Could you check a few things on this model? Use its own coordinates, in mm. A direction names the side the tool comes from. Round coordinates to 2 decimals unless told otherwise and drop trailing zeros. Order: outer loops, then holes, each group sorted by start corner. A loop starts at its lowest first (then second) coordinate and runs counter-clockwise, first axis right, second up. Notation, with made-up numbers: (78.25, 28.25) - (115.25, 28.25) arc R24 cw to (115.25, 39.25) - close; hole circle Ø1 at (52, -20). An arc over 180 degrees is marked (long way). Use one line per item in the form item = value.
from build123d import *

# Parameters (mm, degrees)
CUT_EXTRUDE1_DEPTH      = 269.763771223
CUT_EXTRUDE1_DEPTH_BACK = 269.763771223
CUT_EXTRUDE4_DEPTH      = 13.97
CUT_EXTRUDE5_DEPTH      = 13.97
CIRPATTERN1_COUNT       = 2
CUT_EXTRUDE6_DEPTH      = 269.763771223
CUT_EXTRUDE6_DEPTH_BACK = 269.763771223
FILLET1_R               = 0.254


with BuildPart() as part:
    # Sketch1 → Revolve1 (revolve)
    with BuildSketch(Plane.XY, mode=Mode.PRIVATE) as revolve1_sk:
        with BuildLine():
            Line((-38.8239, 261.4935178), (-43.9039, 261.4935178))
            Line((-43.9039, 261.4935178), (-43.9039, -38.2264822))
            Line((-43.9039, -38.2264822), (-41.2369, -38.2264822))
            Line((-41.2369, -38.2264822), (-41.2369, -52.1964822))
            Line((-41.2369, -52.1964822), (-36.1569, -52.1964822))
            Line((-36.1569, -52.1964822), (-36.1569, -38.2264822))
            ThreePointArc((-36.1569, -38.2264822), (-36.832638636, -32.406611067), (-38.8239, -26.89640228))
            Line((-38.8239, -26.89640228), (-38.8239, 261.4935178))
        make_face()
    revolve(revolve1_sk.sketch.rotate(Axis((0, 16.071963393, 0), (0, -1, 0)), 270), axis=Axis((0, 16.071963393, 0), (0, -1, 0)))

    # Sketch2 → Cut-Extrude1 (cut, two sides: drawn at the far end of the back side and taken through both)
    with BuildSketch(Plane.XY.offset(-CUT_EXTRUDE1_DEPTH_BACK)):
        with BuildLine():
            Line((-0.771031735, -45.62095313), (0, -45.150169247))
            Line((0, -45.150169247), (0.771031735, -45.62095313))
            ThreePointArc((0.771031735, -45.62095313), (0, -48.363269247), (-0.771031735, -45.62095313))
        make_face()
    extrude(amount=CUT_EXTRUDE1_DEPTH + CUT_EXTRUDE1_DEPTH_BACK, mode=Mode.SUBTRACT)

    # Sketch3 → Cut-Extrude4 (cut)
    with BuildSketch(Plane.XZ.offset(52.1964822)):
        with BuildLine():
            Line((-17.427466998, -37.373323583), (0, 0))
            Line((0, 0), (-17.427466998, 37.373323583))
            ThreePointArc((-17.427466998, 37.373323583), (-41.2369, 0), (-17.427466998, -37.373323583))
        make_face()
        with BuildLine():
            Line((17.427466998, 37.373323583), (0, 0))
            Line((0, 0), (17.427466998, -37.373323583))
            ThreePointArc((17.427466998, -37.373323583), (34.778848712, -22.156570219), (41.2369, 0))
            ThreePointArc((41.2369, 0), (34.778848712, 22.156570219), (17.427466998, 37.373323583))
        make_face()
    extrude(amount=-CUT_EXTRUDE4_DEPTH, mode=Mode.SUBTRACT)

    # Sketch4 → Cut-Extrude5 (cut)
    with BuildSketch(Plane.XZ.offset(52.1964822)):
        with BuildLine():
            ThreePointArc((-3.2004, -41.112520738), (-1.601408002, -41.205793452), (0, -41.2369))
            ThreePointArc((0, -41.2369), (1.601408002, -41.205793452), (3.2004, -41.112520738))
            Line((3.2004, -41.112520738), (-3.2004, -41.112520738))
        make_face()
    cut_extrude5 = extrude(amount=-CUT_EXTRUDE5_DEPTH, mode=Mode.SUBTRACT)

    # CirPattern1: Cut-Extrude5 ×2 about axis
    cirpattern1_axis = Axis((0, 0, 0), (0, 1, 0))
    for i in range(1, CIRPATTERN1_COUNT):
        add(cut_extrude5.rotate(cirpattern1_axis, i * 360 / CIRPATTERN1_COUNT), mode=Mode.SUBTRACT)

    # Sketch5 → Cut-Extrude6 (cut, two sides: drawn at the far end of the back side and taken through both)
    with BuildSketch(Plane.XY.offset(-CUT_EXTRUDE6_DEPTH_BACK)):
        with BuildLine():
            Line((-0.771031735, 258.692283917), (0, 259.1630678))
            Line((0, 259.1630678), (0.771031735, 258.692283917))
            ThreePointArc((0.771031735, 258.692283917), (0, 255.9499678), (-0.771031735, 258.692283917))
        make_face()
    extrude(amount=CUT_EXTRUDE6_DEPTH + CUT_EXTRUDE6_DEPTH_BACK, mode=Mode.SUBTRACT)

    # Fillet1
    fillet1_edges = [part.edges().sort_by_distance(p)[0] for p in [
        (-0.385515867, -45.385561188, 41.112520738),
        (0.385515867, -45.385561188, 41.112520738),
        (0, -48.363269247, 41.112520738),
        (0, -48.363269247, -41.112520738),
        (-0.385515867, -45.385561188, -41.112520738),
        (0.385515867, -45.385561188, -41.112520738),
    ]]
    fillet(fillet1_edges, radius=FILLET1_R)


solid = part.part
Item 1: For faces 1 (the face through (-10.38, -45.31, 39.91)), 2 (the face through (10.38, -45.31, -39.91)), 3 (the face through (-11.66, 119.32, 37.03)), 4 (the face through (-0.221, -43.561, -36.156)), 5 (the face through (-10.582, -45.309, -39.856)), which set-ups out of +Z, -Z, +X, -X, +Y, -Y let a thin tool reach every point of the face, with its end or its side?
Found:
face_1 = +Z, -X, -Y
face_2 = -Z, +X, -Y
face_3 = +Y
face_4 = +Y, -Y
face_5 = -Z, -X, -Y
Item 2: Imagine slicing it at B-B on y = 68. Please give me the cut outline in (x, z).
Found:
outline = circle Ø87.81 at (0, 0); hole circle Ø77.65 at (0, 0)
Item 3: If we mould it in two halves opening along Z, with no side actions, what happens to faces 6 (the face through (-1, -45, 41.113)), 7 (the face through (42.86, 109.54, -9.52)), 8 (the face through (0.221, -43.561, 36.156))? For each: released by +Z, released by -Z, zero draft, split by the parting line, or undercut.
Found:
face_6 = released by +Z
face_7 = split by the parting line
face_8 = undercut
Item 4: Imagine slicing it at A-A on z = 0. Please give me the cut outline in (x, y), plus the area to 3 significant figures.
Found:
outline = (-43.9, -38.23) - (-36.16, -38.23) arc R25.4 ccw to (-38.82, -26.9) - (-38.82, 261.49) - (-43.9, 261.49) - close; (36.16, -38.23) - (43.9, -38.23) - (43.9, 261.49) - (38.82, 261.49) - (38.82, -26.9) arc R25.4 ccw to start
area = 3,090 mm2
Item 5: I need wall thicknesses on L1, parallel to Y at x = 0, z = -39.65; L2, parallel to Y at x = 0, z = -42.3; L3, parallel to X at y = 197.5, z = -3. Which ranges of each line are inside material? Lowest first, please.
Found:
L1 = -52.2 to -48.36, -45.15 to 255.95, 259.16 to 261.49
L2 = -38.23 to 255.95, 259.16 to 261.49
L3 = -43.8 to -38.71, 38.71 to 43.8
Item 6: Will these pins go through, and if not, where does the flat tip stop? P1, Ø6, axis at y = 163.5, z = 20.5, coming from the +X side; P2, Ø5, axis at x = -26, y = 186.5, coming from the +Z side; P3, Ø6, axis at y = 199.5, z = 7, coming from the -X side.
Found:
P1 = 40.27
P2 = 37.09
P3 = -43.72
